```python
from build123d import *

# Parameters (mm, degrees)
F0_W     = 95.8645157516
F0_H     = 51.2506449595
F1_DEPTH = 25.4
F2_R     = 33.0176630578
F2_R_2   = 20.4366091001
F3_DEPTH = 42.926
F4_DEPTH = 25.4
F5_DEPTH = 26.67
F7_DEPTH = 30.988
F9_DEPTH = 69.596


with BuildPart() as f1:
    # F0 (on Top) → F1 (new body)
    with BuildSketch(Plane.XY):
        with Locations((0.4608873278, 12.4439517967)):
            Rectangle(F0_W, F0_H)
    extrude(amount=F1_DEPTH)

    # F2 (on face) → F3 (join)
    with BuildSketch(Plane.XY.offset(25.4)):
        with Locations((46.7587672174, 13.9568671584)):
            Circle(F2_R)
        with Locations((46.7587672174, 13.9568671584)):
            Circle(F2_R_2, mode=Mode.SUBTRACT)
    extrude(amount=F3_DEPTH)

    # F4 (add): a face of the model
    f4_faces = [f1.faces().sort_by_distance(p)[0] for p in [
        (61.6753891644, -14.5284210857, 25.4),
    ]]
    extrude(f4_faces, amount=F4_DEPTH)

    # F5 (cut): a face of the model
    f5_faces = [f1.faces().sort_by_distance(p)[0] for p in [
        (38.9613968277, 13.9568671584, 25.4),
    ]]
    extrude(f5_faces, amount=-F5_DEPTH, mode=Mode.SUBTRACT)

    # F6 (on face) → F7 (join)
    with BuildSketch(Plane.XY.offset(25.4)):
        with BuildLine():
            Line((-24.5569236669, 16.9090367761), (-24.5569236669, 7.1940356866))
            Line((-24.5569236669, 7.1940356866), (14.4411221256, 7.1940356866))
            ThreePointArc((14.4411221256, 7.1940356866), (13.797347404, 12.0305033086), (13.8733484372, 16.9090367761))
            Line((13.8733484372, 16.9090367761), (-24.5569236669, 16.9090367761))
        make_face()
    extrude(amount=F7_DEPTH)

    # F8 (on face) → F9 (cut)
    with BuildSketch(Plane.XZ.offset(-7.1940356866)):
        Polygon((-24.5569236669, 56.388), (-24.5569236669, 25.4), (14.4411221256, 56.388), align=None)
    extrude(amount=-F9_DEPTH, mode=Mode.SUBTRACT)


solid = f1.part
```
Geometry: final body of the model. Coordinates: model frame, mm. A direction names the side the tool comes from. Coordinates: 2 decimals unless noted, no trailing zeros. Write each loop counter-clockwise with the first axis right and the second up, starting at its lowest first coordinate (ties: lowest second). Pieces come first, ordered by that corner, then holes. Notation, with made-up numbers: M 24.25,75.25 L 68.25,75.25 A17 ccw 68.25,86.25 Z; hole C -31,-13 d4. An arc over 180 degrees is marked long. Use CSV: the item, a comma, the result in double quotes. Start each with the question number.
1. First-contact query: P1, Ø12, axis at x = 58.5, z = 56, coming from the -Y side; P2, Ø3, axis at x = 9.5, z = 43.5, coming from the -Y side; P3, Ø9, axis at x = -1, z = 38.5, coming from the +Y side; P4, Ø0.8, axis at x = 14, y = 11.5, coming from the -Z side. Flat tips, straight axial feed; report the tip coordinate or a pass-through.
2. Cut plane D-D on x = -1. Return the cut outline in (y, z), plus the area to 3 significant figures.
3. Cut plane C-C on y = 8.5. Return the cut outline in (x, z).
4. Ray query, probe 1 along Z at (x, y) = (-21, 4); probe 2 along Y at (x, z) = (-17, 27); probe 3 along Y at (x, z) = (-31, 11.5). Return the intervals inside material, ascending.
5. Reachability of faces 1 (the face through (3, 7.194, 34)), 2 (the face through (-12, 38.069, 13)), 3 (the face through (-1, 16.909, 37)) from +Z, -Z, +X, -X, +Y, -Y: full face, straight path, thin tool, end or side. Return the list, or none.
6. Cut plane B-B on z = 14.5. Return the cut outline in (x, y).
7. Cut plane A-A on x = 59. Return the cut outline in (y, z).
Entries:
1,P1,"y = -18.56"
1,P2,"y = 7.19"
1,P3,"y = 16.91"
1,P4,"z = 0"
2,outline,"M -13.18,0 L 38.07,0 L 38.07,25.4 L 16.91,25.4 L 16.91,44.12 L 7.19,44.12 L 7.19,25.4 L -13.18,25.4 Z"
2,area,"1,480 mm²"
3,outline,"M -47.47,0 L 27.06,0 L 27.06,68.33 L 14.2,68.33 L 14.2,56.39 L 14.44,56.39 L -24.56,25.4 L -47.47,25.4 Z; M 66.45,0 L 79.32,0 L 79.32,68.33 L 66.45,68.33 Z"
4,probe 1,"0 to 25.4"
4,probe 2,"7.19 to 16.91"
4,probe 3,"-13.18 to 38.07"
5,face 1,"+Z, -X, -Y"
5,face 2,"+Z, -Z, -X, +Y"
5,face 3,"+Z, -X, +Y"
6,outline,"M -47.47,-13.18 L 27.95,-13.18 A33.02 ccw long 24.2,38.07 L -47.47,38.07 Z; hole C 46.76,13.96 d40.87"
7,outline,"M -16.71,0 L -2.41,0 L -2.41,68.33 L -16.71,68.33 Z; M 30.32,0 L 44.62,0 L 44.62,68.33 L 30.32,68.33 Z"
